Part model, mm, in its own coordinate system. Face numbers are marked on the shaded views. Round coordinates to 2 decimals unless told otherwise and drop trailing zeros.
(1) Mould opens along Z. For the marked faces 1 and 2 say: +Z half, -Z half, draft (parallel to the pull), parting line (faces both ways), or undercut.
(2) Probe probe 1 along X at (y, z) = (-103, 3.4); probe 2 along Y at (x, z) = (-50, 3.15). List the from-to ranges inside material, lowest first.
(3) Flat gauge pin, fed straight in: pin 1 (5.5 mm diameter, centred on x = -50, y = -103, fed in from -Z). Where does the tip first touch, or does it go through?
Autodesk Inventor part; units mm, degrees
ref_plane "YZ Plane" through (0, 0, 0) normal (1, 0, 0) x (0, 1, 0)
ref_plane "XZ Plane" through (0, 0, 0) normal (0, 1, 0) x (-1, 0, 0)
ref_plane "XY Plane" through (0, 0, 0) normal (0, 0, 1) x (1, 0, 0)
sketch "Sketch1" plane through (0, 0, 0) normal (0, 0, 1) x (1, 0, 0)
  line L0 (-70, -115) -> (70, -115)
  line L1 (70, -115) -> (70, 115)
  line L2 (70, 115) -> (-70, 115)
  line L3 (-70, 115) -> (-70, -115)
  point P0 (0, 0)
  dimension "width" = 140
  dimension "d1" = 70
  dimension "d2" = 230
  dimension "d3" = 115
extrude "Extrusion1" add sketch "Sketch1" along normal blind 5
sketch "Sketch3" plane through (0, 0, 5) normal (0, 0, 1) x (1, 0, 0)
  line L0 (-70, 115) -> (-70, -115)
  line L1 (-70, -115) -> (70, -115)
  point P0 (0, 0)
  point P1 (-50, -103)
  point P2 (50, -103)
  dimension "d33" = 20
  dimension "d34" = 12
  dimension "d35" = 12
  dimension "d36" = 20
hole "Hole1" at (-50, -103, 5) at (50, -103, 5) direction (0, 0, -1) diameter 3.5 end through all
properties part number "EBF_005.1-bottom-plate_cup-holder"
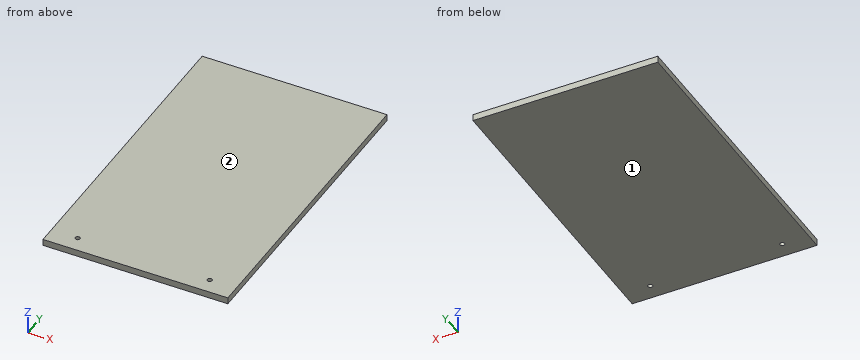
Final values:
1. face 1: -Z half
1. face 2: +Z half
2. probe 1: x = -70 to -51.75, -48.25 to 48.25, 51.75 to 70
2. probe 2: y = -115 to -104.75, -101.25 to 115
3. pin 1: stops at z = 0
